Check sheet for the modelled part. Datum: model origin and axes. Units: mm. A direction names the side the tool comes from. Round coordinates to 2 decimals unless told otherwise and drop trailing zeros. Write each loop counter-clockwise with the first axis right and the second up, starting at its lowest first coordinate (ties: lowest second). Pieces come first, ordered by that corner, then holes.
Item 1: Material ranges on line 1 (Y direction, x = 0.5, z = 1.7); line 2 (Y direction, x = -5, z = 0.85); line 3 (Z direction, x = 1.5, y = -1), recorded low to high.
Item 2: Cross-section at C-C on z = 0.95. Enter the section's corners in (x, y).
Item 3: Cross-section at A-A on y = 5. Enter the section's corners in (x, z).
Item 4: Cross-section at D-D on y = 0. Enter the section's corners in (x, z).
Item 5: Tool access check on faces 5 (the flat face through (-15, -17, 6)), 6 (the flat face through (0, 0, 0)), 7 (the flat face through (9, -16, 5)), 8 (the flat face through (12.2, 17, 3)), 9 (the flat face through (-12.853, 17, 4)). Record the directions out of +Z, -Z, +X, -X, +Y, -Y that give a thin tool (end or side, any length) a straight path to the whole face; none if there is none.
Item 6: Go/stop test with flat-tipped pins: pin 1 Ø1.6 at (y, z) = (-16.5, 5) entering from -X; pin 2 Ø2 at (x, z) = (-1, 4) entering from -Y; pin 3 Ø3.5 at (x, y) = (5, 0) entering from -Z; pin 4 Ø5 at (x, y) = (0, -5) entering from +Z. Record where each tip stops, or that it passes through.
Item 7: Release check for a two-part mould opening along X. For faces 1 (the cylindrical face through (-10.99, 17.01, 4.76)), 2 (the flat face through (-12.25, -17, 4)), 3 (the flat face through (-1, 16, 4)), 4 (the flat face through (-17.5, 0, 1)) record: +X half, -X half, draft (parallel to the pull), parting line (faces both ways), or undercut.
Item 8: Cross-section at B-B on x = -14.5. Enter the section's corners in (y, z).
from build123d import *

# Parameters (mm, degrees)
CROQUIS1_W              = 36
CROQUIS1_H              = 35
CROQUIS1_R              = 2
SALIENTE_EXTRUIR1_DEPTH = 2
CROQUIS2_R              = 1.25
SALIENTE_EXTRUIR2_DEPTH = 2
SALIENTE_EXTRUIR3_START = -2
CROQUIS3_W              = 4.5
CROQUIS3_H              = 6
CROQUIS3_R              = 1.25140183
CROQUIS3_R_2            = 1.25
SALIENTE_EXTRUIR3_DEPTH = 2


with BuildPart() as part:
    # Croquis1 → Saliente-Extruir1 (new body)
    with BuildSketch(Plane(origin=(0, 0, 0), x_dir=(0, 1, 0), z_dir=(0, 0, 1))):
        Rectangle(CROQUIS1_W, CROQUIS1_H)
        with Locations(Location((0, 5, 0), (0, 0, 270))):
            Circle(CROQUIS1_R, mode=Mode.SUBTRACT)
        with Locations(Location((5, 0, 0), (0, 0, 270))):
            Circle(CROQUIS1_R, mode=Mode.SUBTRACT)
        with Locations(Location((0, -5, 0), (0, 0, 270))):
            Circle(CROQUIS1_R, mode=Mode.SUBTRACT)
        with Locations(Location((-5, 0, 0), (0, 0, 270))):
            Circle(CROQUIS1_R, mode=Mode.SUBTRACT)
    extrude(amount=SALIENTE_EXTRUIR1_DEPTH)

    # Croquis2 → Saliente-Extruir2 (add)
    with BuildSketch(Plane(origin=(0, 18, 0), x_dir=(-1, 0, 0), z_dir=(0, 1, 0))):
        Polygon((-10.95, 6), (12.85345456, 6), (12.85345456, 0), (-12.2, 0), (-12.2, 4.75), align=None)
        with Locations((-10, 4)):
            Circle(CROQUIS2_R, mode=Mode.SUBTRACT)
        with Locations(Location((10, 4, 0), (0, 0, 180))):
            Circle(CROQUIS2_R, mode=Mode.SUBTRACT)
    extrude(amount=-SALIENTE_EXTRUIR2_DEPTH)

    # Croquis3 → Saliente-Extruir3 (add)
    # profile 1 of 2: a face of its own
    with BuildSketch(Plane.XZ.offset(18).offset(SALIENTE_EXTRUIR3_START)):
        with Locations((-14.5, 3)):
            Rectangle(CROQUIS3_W, CROQUIS3_H)
        with Locations((-14.5, 4)):
            Circle(CROQUIS3_R, mode=Mode.SUBTRACT)
    # profile 2 of 2: a face of its own
    with BuildSketch(Plane.XZ.offset(18).offset(SALIENTE_EXTRUIR3_START)):
        Polygon((12.2, 4.75), (10.95, 6), (8, 6), (8, 2), (12.2, 2), align=None)
        with Locations(Location((10, 4, 0), (0, 0, 180))):
            Circle(CROQUIS3_R_2, mode=Mode.SUBTRACT)
    extrude(amount=SALIENTE_EXTRUIR3_DEPTH)


solid = part.part
Response values:
1. line 1: y = -18 to -6.94, -3.06 to 3.06, 6.94 to 18
1. line 2: y = -18 to -2, 2 to 18
1. line 3: z = 0 to 2
2. outline: (-17.5, -18) - (17.5, -18) - (17.5, 18) - (-17.5, 18) - close; hole circle Ø4 at (-5, 0); hole circle Ø4 at (0, -5); hole circle Ø4 at (0, 5); hole circle Ø4 at (5, 0)
3. outline: (-17.5, 0) - (-2, 0) - (-2, 2) - (-17.5, 2) - close; (2, 0) - (17.5, 0) - (17.5, 2) - (2, 2) - close
4. outline: (-17.5, 0) - (-7, 0) - (-7, 2) - (-17.5, 2) - close; (-3, 0) - (3, 0) - (3, 2) - (-3, 2) - close; (7, 0) - (17.5, 0) - (17.5, 2) - (7, 2) - close
5. face 5: +Z, +X, -X, +Y, -Y
5. face 6: -Z, +X, -X, +Y, -Y
5. face 7: +Z, +X, -X
5. face 8: +Z, +X, +Y, -Y
5. face 9: +Z, -X, +Y
6. pin 1: stops at x = -16.75
6. pin 2: stops at y = 16
6. pin 3: passes through
6. pin 4: stops at z = 2
7. face 1: undercut
7. face 2: undercut
7. face 3: draft
7. face 4: -X half
8. outline: (-18, 0) - (18, 0) - (18, 2) - (-16, 2) - (-16, 2.75) - (-18, 2.75) - close; (-18, 5.25) - (-16, 5.25) - (-16, 6) - (-18, 6) - close
